```python
from build123d import *

# Parameters (mm, degrees)
SKICA1_W                 = 13
SKICA1_H                 = 23.5
P_IDAT_VYSUNUT_M1_DEPTH  = 1
SKICA2_W                 = 13
SKICA2_H                 = 1
P_IDAT_VYSUNUT_M2_DEPTH  = 1
SKICA3_R                 = 2
ODEBRAT_VYSUNUT_M1_DEPTH = 1
SKICA4_W                 = 13
SKICA4_H                 = 3.5
ODEBRAT_VYSUNUT_M2_DEPTH = 10


with BuildPart() as part:
    # Skica1 → Přidat vysunutím1 (new body)
    with BuildSketch(Plane.XY):
        with Locations((6.5, 11.75)):
            Rectangle(SKICA1_W, SKICA1_H)
    extrude(amount=P_IDAT_VYSUNUT_M1_DEPTH)

    # Skica2 → Přidat vysunutím2 (add)
    with BuildSketch(Plane.XY.offset(1)):
        with Locations((6.5, 23)):
            Rectangle(SKICA2_W, SKICA2_H)
        with Locations((6.5, 7)):
            Rectangle(SKICA2_W, SKICA2_H)
    extrude(amount=P_IDAT_VYSUNUT_M2_DEPTH)

    # Skica3 → Odebrat vysunutím1 (cut)
    with BuildSketch(Plane.XY.offset(1)):
        with Locations((6.5, 15)):
            Circle(SKICA3_R)
    extrude(amount=-ODEBRAT_VYSUNUT_M1_DEPTH, mode=Mode.SUBTRACT)

    # Skica4 → Odebrat vysunutím2 (cut)
    with BuildSketch(Plane.XY.offset(1)):
        with Locations((6.5, 1.75)):
            Rectangle(SKICA4_W, SKICA4_H)
    extrude(amount=-ODEBRAT_VYSUNUT_M2_DEPTH, mode=Mode.SUBTRACT)


solid = part.part
```
Verification items for the finished model (mm, model axes). A direction names the side the tool comes from. Round coordinates to 2 decimals unless told otherwise and drop trailing zeros. Write each loop counter-clockwise with the first axis right and the second up, starting at its lowest first coordinate (ties: lowest second). Pieces come first, ordered by that corner, then holes. Notation, with made-up numbers: (68.5, 86.5) - (75.5, 86.5) arc R10 ccw to (75.5, 91.5) - close; hole circle Ø11 at (-17.75, 53.25). An arc over 180 degrees is marked (long way). Answer as a JSON object with one key per item and string values. Group by question number.
Q1. Go/stop test with flat-tipped pins: pin 1 Ø1.5 at (x, y) = (7.5, 5) entering from +Z; pin 2 Ø2 at (x, y) = (6, 12.5) entering from -Z; pin 3 Ø0.5 at (x, z) = (8.5, 1.5) entering from -Y. Record where each tip stops, or that it passes through.
Q2. Section check D-D, the plane x = 9.5. Enter the section's corners in (y, z).
Q3. Section check A-A, the plane x = 6.5. Enter the section's corners in (y, z).
Q4. Section check C-C, the plane y = 15. Enter the section's corners in (x, z), plus the area to 3 significant figures.
Q5. Thickness scan on line 1 (Y direction, x = 7.75, z = 1.1); line 2 (Y direction, x = 6.5, z = 0.75); line 3 (Z direction, x = 5, y = 6). Record the ranges inside material, lowest first.
Q6. Section check B-B, the plane z = 1.4. Enter the section's corners in (x, y), plus the area to 3 significant figures.
Q7. Tool access check on faces 1 (the flat face through (6, 23, 2)), 2 (the flat face through (6.4, 22.5, 1.5)), 3 (the flat face through (6, 5, 1)). Record the directions out of +Z, -Z, +X, -X, +Y, -Y that give a thin tool (end or side, any length) a straight path to the whole face; none if there is none.
Q8. Mould release check, pull along Y, two halves, no side actions. Record for faces 4 (the flat face through (6, 7, 2)), 5 (the flat face through (8, 17, 1)), 6 (the flat face through (6.4, 6.5, 1.5)): released by +Y, released by -Y, zero draft, split by the parting line, or undercut.
Found:
{
 "1": {"pin 1": "stops at z = 1", "pin 2": "stops at z = 0", "pin 3": "stops at y = 6.5"},
 "2": {"outline": "(3.5, 0) - (23.5, 0) - (23.5, 2) - (22.5, 2) - (22.5, 1) - (7.5, 1) - (7.5, 2) - (6.5, 2) - (6.5, 1) - (3.5, 1) - close"},
 "3": {"outline": "(3.5, 0) - (13, 0) - (13, 1) - (7.5, 1) - (7.5, 2) - (6.5, 2) - (6.5, 1) - (3.5, 1) - close; (17, 0) - (23.5, 0) - (23.5, 2) - (22.5, 2) - (22.5, 1) - (17, 1) - close"},
 "4": {"outline": "(0, 0) - (4.5, 0) - (4.5, 1) - (0, 1) - close; (8.5, 0) - (13, 0) - (13, 1) - (8.5, 1) - close", "area": "9.00 mm^2"},
 "5": {"line 1": "y = 6.5 to 7.5, 22.5 to 23.5", "line 2": "y = 3.5 to 13, 17 to 23.5", "line 3": "z = 0 to 1"},
 "6": {"outline": "(0, 6.5) - (13, 6.5) - (13, 7.5) - (0, 7.5) - close; (0, 22.5) - (13, 22.5) - (13, 23.5) - (0, 23.5) - close", "area": "26.0 mm^2"},
 "7": {"face 1": "+Z, +X, -X, +Y, -Y", "face 2": "+Z, +X, -X", "face 3": "+Z, +X, -X, -Y"},
 "8": {"face 4": "zero draft", "face 5": "undercut", "face 6": "released by -Y"}
}
